Autodesk Inventor part; units mm, degrees
ref_plane "YZ Plane" through (0, 0, 0) normal (1, 0, 0) x (0, 1, 0)
ref_plane "XZ Plane" through (0, 0, 0) normal (0, 1, 0) x (-1, 0, 0)
ref_plane "XY Plane" through (0, 0, 0) normal (0, 0, 1) x (1, 0, 0)
sketch "Boceto1" plane through (0, 0, 0) normal (0, 1, 0) x (-1, 0, 0)
  circle A0 centre (0, 0) radius 13
  dimension "d0" = 26
extrude "Extrusión1" add sketch "Boceto1" along normal blind 151
sketch "Boceto2" plane through (0, 151, 0) normal (0, 1, 0) x (1, 0, 0)
  circle A0 centre (0, 0) radius 10.75
  circle A1 centre (0, 0) radius 13
  dimension "d3" = 21.5
extrude "Extrusión2" cut sketch "Boceto2" against normal blind 37.2
fillet "Empalme1" radius 6 1 edges at (-10.75, 151, 0)
thread "Rosca1"
sketch "Boceto3" plane through (0, 0, 0) normal (0, -1, 0) x (1, 0, 0)
  circle A0 centre (0, 0) radius 6.5
  circle A1 centre (0, 0) radius 13
  dimension "d9" = 13
extrude "Extrusión3" cut sketch "Boceto3" against normal blind 10
sketch "Boceto4" plane through (0, 10, 0) normal (0, -1, 0) x (1, 0, 0)
  circle A0 centre (0, 0) radius 13
  circle A1 centre (0, 0) radius 12.95
  dimension "d12" = 25.9
extrude "Extrusión4" cut sketch "Boceto4" against normal blind 20
thread "Rosca2"
thread "Rosca3"
properties part number "W504"
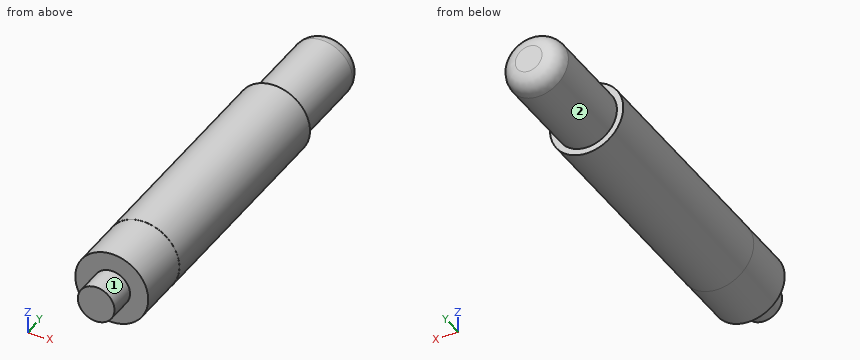
CAD build for the part. Positions are in the model's coordinates, mm. Face numbers are marked on the shaded views. A direction names the side the tool comes from. Round coordinates to 2 decimals unless told otherwise and drop trailing zeros. Write each loop counter-clockwise with the first axis right and the second up, starting at its lowest first coordinate (ties: lowest second). Pieces come first, ordered by that corner, then holes.
(1) 3-axis set-ups, long thin cutter, end or side, ignore diameter. For the marked faces 1 and 2: which of +Z, -Z, +X, -X, +Y, -Y reach the whole face in a straight line?
(2) Probe line 1 along Z through (x, y) = (0.25, 41); line 2 along Y through (x, z) = (5, 11.25); line 3 along X through (y, z) = (79.5, 7.75). List the from-to ranges inside material, lowest first.
(3) Slice it at A-A, the plane y = 68.5. Write the cut outline in (x, z), and give its area (3 significant figures).
(4) Drop flat-ended pins along their axis: P1, Ø6, axis at x = 1.5, z = -10, coming from the -Y side; P2, Ø4, axis at x = 7, y = 39, coming from the +Z side; P3, Ø5, axis at x = 5, z = -8.5, coming from the +Y side. Give the stop position or say it passes through.
From the geometry:
1. face 1: -Y
1. face 2: +Y
2. line 1: z = -13 to 13
2. line 2: y = 10 to 113.8
2. line 3: x = -10.44 to 10.44
3. outline: circle Ø26 at (0, 0)
3. area: 531 mm2
4. P1: stops at y = 10
4. P2: stops at z = 12
4. P3: stops at y = 150.4
